Design review of the part shown in the three views and the two pictorial views. Dimensions are in mm from the part's minimum x, y and z. A direction names the side the tool comes from. Round coordinates to 2 decimals unless told otherwise and drop trailing zeros. Order: outer loops, then holes, each group sorted by start corner. A loop starts at its lowest first (then second) coordinate and runs counter-clockwise, first axis right, second up.
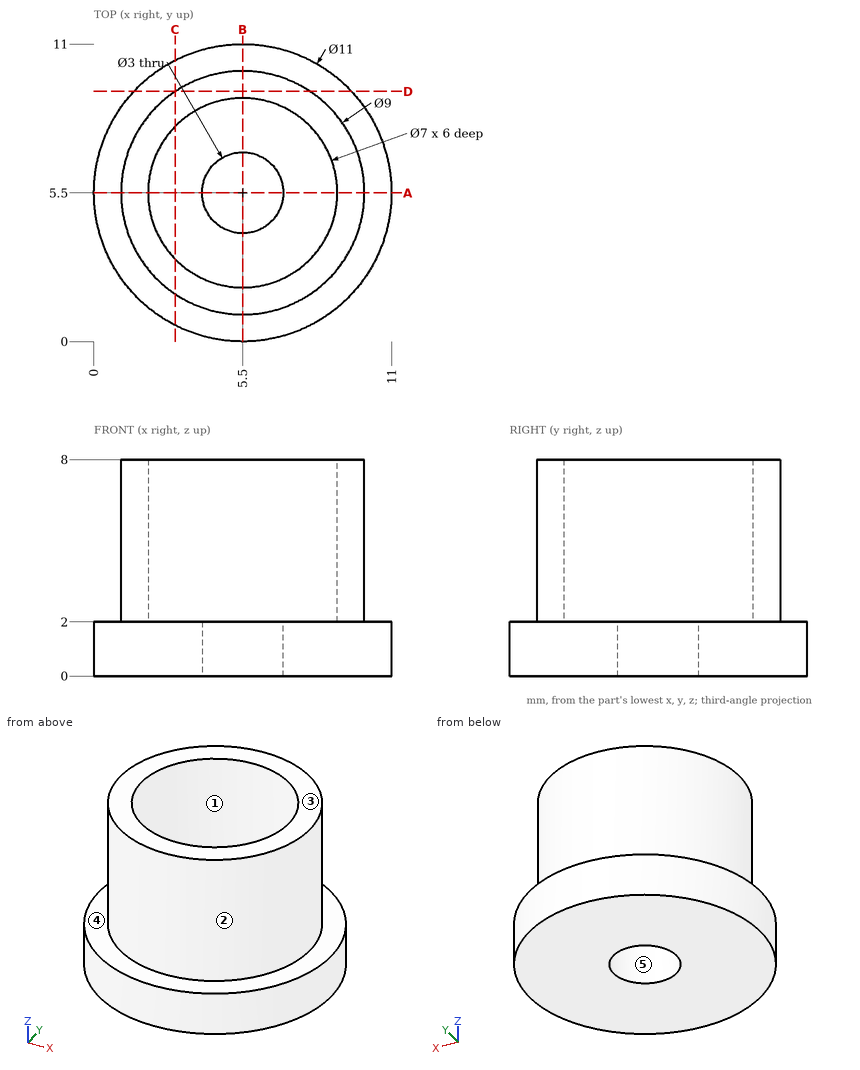
1) Take a section at A-A on y = 5.5. Give the boundary of the cut face in (x, z).
Results:
outline: (0, 0) - (4, 0) - (4, 2) - (2, 2) - (2, 8) - (1, 8) - (1, 2) - (0, 2) - close; (7, 0) - (11, 0) - (11, 2) - (10, 2) - (10, 8) - (9, 8) - (9, 2) - (7, 2) - close
2) The part is to be moulded in two halves that separate along Y. For the marked faces 1, 2 and 3, say which applies: released by +Y, released by -Y, zero draft, split by the parting line, or undercut.
Results:
face 1: undercut
face 2: split by the parting line
face 3: zero draft
3) To check wall thickness, follow line 1 along Y through (x, z) = (5.5, 5.9); line 2 along Y through (x, z) = (5.5, 0.8); line 3 along Z through (x, y) = (7.25, 8). State the ranges of each line that lie inside material, in increasing order.
Results:
line 1: y = 1 to 2, 9 to 10
line 2: y = 0 to 4, 7 to 11
line 3: z = 0 to 2
4) Take a section at C-C on x = 3. Give the boundary of the cut face in (y, z).
Results:
outline: (0.6, 0) - (10.4, 0) - (10.4, 2) - (9.24, 2) - (9.24, 8) - (7.95, 8) - (7.95, 2) - (3.05, 2) - (3.05, 8) - (1.76, 8) - (1.76, 2) - (0.6, 2) - close
5) Take a section at D-D on y = 9.25. Give the boundary of the cut face in (x, z), plus the area to 3 significant figures.
Results:
outline: (1.48, 0) - (9.52, 0) - (9.52, 2) - (7.99, 2) - (7.99, 8) - (3.01, 8) - (3.01, 2) - (1.48, 2) - close
area: 45.9 mm2
6) For the marked faces 4 and 5, list the 3-axis set-ups (+Z, -Z, +X, -X, +Y, -Y) from which the entire face can be reached by the end or side of a thin tool; tool diameter is ignored.
Results:
face 4: +Z
face 5: +Z, -Z
7) Clearance check with flat-ended pins moving along their axes: P1, Ø2, axis at y = 10, z = 6, coming from the +X side; P2, Ø4, axis at x = 8.5, z = 4.5, coming from the +Y side; P3, Ø5.5, axis at x = 5.5, y = 5.5, coming from the +Z side; P4, Ø2.5, axis at x = 5.5, y = 5.5, coming from the -Z side. State where each tip first meets the part, or that it passes through.
Results:
P1: stops at x = 8.33
P2: stops at y = 9.89
P3: stops at z = 2
P4: passes through
